from build123d import *

# Parameters (mm, degrees)
F0_W     = 75
F0_H     = 25
F0_W_2   = 69
F0_H_2   = 17
F1_DEPTH = 45
F2_W     = 39
F2_H     = 17
F3_DEPTH = 100
F5_START = 4
F4_W     = 142
F4_H     = 82
F5_DEPTH = 26


with BuildPart() as f1:
    # F0 (on Front) → F1 (new body, symmetric)
    with BuildSketch(Plane.XZ):
        with Locations((-37.5, 12.5)):
            Rectangle(F0_W, F0_H)
        with Locations((-36.5, 12.5)):
            Rectangle(F0_W_2, F0_H_2, mode=Mode.SUBTRACT)
        with Locations((37.5, 12.5)):
            Rectangle(F0_W, F0_H)
        with Locations((36.5, 12.5)):
            Rectangle(F0_W_2, F0_H_2, mode=Mode.SUBTRACT)
    extrude(amount=F1_DEPTH, both=True)

    # F2 (on Right) → F3 (cut, symmetric)
    with BuildSketch(Plane.YZ):
        with Locations((21.5, 12.5)):
            Rectangle(F2_W, F2_H)
        with Locations((-21.5, 12.5)):
            Rectangle(F2_W, F2_H)
    extrude(amount=F3_DEPTH, both=True, mode=Mode.SUBTRACT)

    # F4 (on Top) → F5 (cut)
    with BuildSketch(Plane.XY.offset(F5_START)):
        Rectangle(F4_W, F4_H)
    extrude(amount=F5_DEPTH, mode=Mode.SUBTRACT)


solid = f1.part
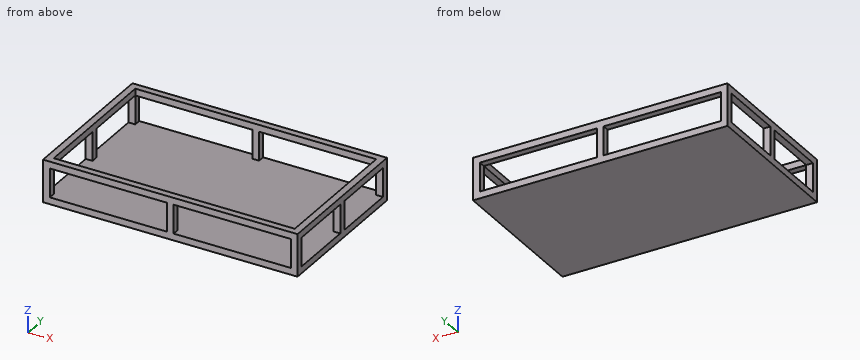
Geometry: final body of the model. Coordinates: model frame, mm. Round coordinates to 2 decimals unless told otherwise and drop trailing zeros. Loops run counter-clockwise (first coordinate to the right, second up) from the corner with the lowest first, then second, coordinate; pieces in that order, holes last. Notation, with made-up numbers: M 74.25,87 L 100.25,87 A24 cw 100.25,97 Z; hole C 42,10.25 d8. An arc over 180 degrees is marked long. Put each result on its own line as item: value. Start each with the question number.
(1) Contact query for a flat-ended pin moving along its axis: pin 1 Ø4 at (x, y) = (49.5, 33) entering from +Z. Output: stop coordinate, or through.
(2) Material intervals for line 1 along Y through (x, z) = (-62, 23.25); line 2 along X through (y, z) = (-3, 22.5); line 3 along Z through (x, y) = (52.5, 15), sorted ascending. Write a range as [from, to].
(3) Section query C-C (x = -26). Return loops of the section in (y, z).
(4) Section query B-B (y = 32). Return loops of the section in (x, z), then the cut area to 3 significant figures.
(5) Section query A-A (z = 9.25). State how many separate pieces and enclosed holes the cut face has, then the cut area to 3 significant figures.
Findings below:
1. pin 1: stops at z = 4
2. line 1: y = [-45, -41], [41, 45]
2. line 2: x = [-75, -71], [71, 75]
2. line 3: z = [0, 4]
3. outline: M -45,0 L 45,0 L 45,4 L -45,4 Z; M -45,21 L -41,21 L -41,25 L -45,25 Z; M 41,21 L 45,21 L 45,25 L 41,25 Z
4. outline: M -75,0 L 75,0 L 75,4 L -75,4 Z; M -75,21 L -71,21 L -71,25 L -75,25 Z; M 71,21 L 75,21 L 75,25 L 71,25 Z
4. area: 632 mm2
5. separate pieces: 8
5. enclosed holes: 0
5. area: 128 mm2
